from build123d import *

# Parameters (mm, degrees)
BOSS_EXTRUDE1_DEPTH = 5
FILLET1_R           = 10
FILLET2_R           = 10


with BuildPart() as part:
    # Sketch1 → Boss-Extrude1 (new body)
    with BuildSketch(Plane.XY):
        with BuildLine():
            Line((-5, 0), (-5, 15))
            Line((-5, 15), (7, 30.096250941))
            Line((7, 30.096250941), (7, 40))
            Line((7, 40), (10, 40))
            Line((10, 40), (10, 30))
            Line((10, 30), (5, 15))
            Line((5, 15), (5, 0))
            ThreePointArc((5, 0), (0, -5), (-5, 0))
        make_face()
        with BuildLine():
            Line((-1.193733639, 1.175), (1.193733639, 1.175))
            ThreePointArc((1.193733639, 1.175), (0, -1.675), (-1.193733639, 1.175))
        make_face(mode=Mode.SUBTRACT)
    extrude(amount=BOSS_EXTRUDE1_DEPTH)

    # Fillet1
    fillet1_edges = [part.edges().sort_by_distance(p)[0] for p in [
        (-5, 15, 2.5),
        (10, 30, 2.5),
    ]]
    fillet(fillet1_edges, radius=FILLET1_R)

    # Fillet2
    fillet2_edges = [part.edges().sort_by_distance(p)[0] for p in [
        (7, 30.096250941, 2.5),
        (5, 15, 2.5),
    ]]
    fillet(fillet2_edges, radius=FILLET2_R)


solid = part.part
Input: part model. Units: mm. Frame: model coordinates. A direction names the side the tool comes from. Give positions to 0.01 mm unless a question says otherwise; leave off trailing zeros. Order: outer loops, then holes, each group sorted by start corner. A loop starts at its lowest first (then second) coordinate and runs counter-clockwise, first axis right, second up. Notation, with made-up numbers: M -21,59.25 L 9,59.25 A31 cw 9,97.25 Z; hole C -27,-3 d10. An arc over 180 degrees is marked long. Answer as a JSON object with one key per item and string values.
1. Ray query, line 1 (X direction, y = 0, z = 1.55) (3 decimals); line 2 (X direction, y = 34.5, z = 3.4); line 3 (Y direction, x = 1.25, z = 2.5). Return the intervals inside material, ascending. Write a range as [from, to].
Result sheet:
{"line 1": "[-5, -1.675], [1.675, 5]", "line 2": "[7, 10]", "line 3": "[-4.84, -1.11], [1.11, 22.86]"}
2. Cut plane C-C, the plane y = 10. Output: boundary loops of the cut face in (x, z), and give its area (3 significant figures).
Result sheet:
{"outline": "M -5,0 L 5,0 L 5,5 L -5,5 Z", "area": "50.0 mm²"}
3. Cut plane B-B, the plane x = 0. Output: boundary loops of the cut face in (y, z) (3 decimals), and give its area (3 significant figures).
Result sheet:
{"outline": "M -5,0 L -1.675,0 L -1.675,5 L -5,5 Z; M 1.175,0 L 21.29,0 L 21.29,5 L 1.175,5 Z", "area": "117 mm²"}
4. Reachability of faces 5 (the flat face through (5, 7, 2)), 6 (the flat face through (7, 37, 2)), 7 (the flat face through (3, 13, 0)) from +Z, -Z, +X, -X, +Y, -Y: full face, straight path, thin tool, end or side. Return the list, or none.
Result sheet:
{"face 5": "+Z, -Z, +X, -Y", "face 6": "+Z, -Z, -X, +Y", "face 7": "-Z, +X, -X, +Y, -Y"}
5. Pull-direction query (X, two-part tool) for faces 1 (the cylindrical face through (9.867, 29.999, 2.535)), 2 (the flat face through (0, 1.175, 2)), 3 (the cylindrical face through (-4.457, 14.761, 2.535)), 4 (the flat face through (3, 13, 5)); classes: +X half, -X half, draft (parallel to the pull), parting line (faces both ways), or undercut.
Result sheet:
{"face 1": "+X half", "face 2": "undercut", "face 3": "-X half", "face 4": "draft"}
6. Cut plane D-D, the plane x = 6.5. Output: boundary loops of the cut face in (y, z), and give its area (3 significant figures).
Result sheet:
{"outline": "M 19.5,0 L 30.46,0 L 30.46,5 L 19.5,5 Z", "area": "54.8 mm²"}
7. First-contact query: P1, Ø1.5, axis at y = 3.5, z = 3, coming from the +X side; P2, Ø1.5, axis at y = 36, z = 3, coming from the -X side; P3, Ø2, axis at x = 0, y = 0, coming from the -Z side; P4, Ø3, axis at x = -3.5, z = 2.5, coming from the -Y side. Flat tips, straight axial feed; report the tip coordinate or a pass-through.
Result sheet:
{"P1": "x = 5", "P2": "x = 7", "P3": "through", "P4": "y = -4.58"}
